from build123d import *

# Parameters (mm, degrees)
SKETCH1_W           = 25.4
SKETCH1_H           = 38.1
BOSS_EXTRUDE1_DEPTH = 609.6
SHELL1_T            = -3.175
SKETCH2_R           = 2.38125
CUT_EXTRUDE1_DEPTH  = 611.426262951


with BuildPart() as part:
    # Sketch1 → Boss-Extrude1 (new body)
    with BuildSketch(Plane.XY):
        Rectangle(SKETCH1_W, SKETCH1_H)
    extrude(amount=BOSS_EXTRUDE1_DEPTH)

    # Shell1
    shell1_openings = [part.faces().sort_by_distance(p)[0] for p in [
        (0, 0, 609.6),
        (0, 0, 0),
    ]]
    offset(amount=SHELL1_T, openings=shell1_openings, kind=Kind.INTERSECTION)

    # Sketch2 → Cut-Extrude1 (cut, through all)
    with BuildSketch(Plane(origin=(12.7, 0, 0), x_dir=(0, 0, -1), z_dir=(1, 0, 0))):
        with Locations(Location((-44.45, 6.35, 0), (0, 0, 90))):
            Circle(SKETCH2_R)
        with Locations(Location((-63.5, 6.35, 0), (0, 0, 90))):
            Circle(SKETCH2_R)
    extrude(amount=-CUT_EXTRUDE1_DEPTH, mode=Mode.SUBTRACT)


solid = part.part
Verification items for the finished model (mm, model axes). A direction names the side the tool comes from. Round coordinates to 2 decimals unless told otherwise and drop trailing zeros. Loops run counter-clockwise (first coordinate to the right, second up) from the corner with the lowest first, then second, coordinate; pieces in that order, holes last. Notation, with made-up numbers: (44, 22) - (90, 22) arc R24 ccw to (90, 50) - close; hole circle Ø9 at (89.5, 7). An arc over 180 degrees is marked (long way). Use a Markdown table: item, result. Add a question column.
1. Access from +Z, -Z, +X, -X, +Y, -Y to the whole of each face (thin tool, end or side, straight path). Record for faces 4 (the face through (-9.525, 0, 301)), 5 (the face through (12.7, 0, 301)).
2. Section check A-A, the plane x = -1.75. Record the boundary of the cut face in (y, z) (3 decimals).
3. Thickness scan on probe 1 along Z at (x, y) = (-11.15, 6.35); probe 2 along Y at (x, z) = (-1, 365.5) (3 decimals); probe 3 along X at (y, z) = (-0.5, 467) (3 decimals). Record the ranges inside material, lowest first. Write a range as [from, to].
4. Release check for a two-part mould opening along Y. For faces 1 (the face through (0, 15.875, 301)), 2 (the face through (0, 19.05, 301)), 3 (the face through (11, 0, 0)) record: released by +Y, released by -Y, zero draft, split by the parting line, or undercut.
5. Section check B-B, the plane z = 115. Record the boundary of the cut face in (x, y) (3 decimals).
6. Gauge pin test, flat end, axial feed: pin 1 (5.5 mm diameter, centred on y = 6.35, z = 44.45, fed in from +X). Record the tip position at first contact, or that the pin passes through.
Checks:
| question | item | result |
|---|---|---|
| 1 | face 4 | +Z, -Z |
| 1 | face 5 | +Z, -Z, +X, +Y, -Y |
| 2 | outline | (-19.05, 0) - (-15.875, 0) - (-15.875, 609.6) - (-19.05, 609.6) - close; (15.875, 0) - (19.05, 0) - (19.05, 609.6) - (15.875, 609.6) - close |
| 3 | probe 1 | z = [0, 42.07], [46.83, 61.12], [65.88, 609.6] |
| 3 | probe 2 | y = [-19.05, -15.875], [15.875, 19.05] |
| 3 | probe 3 | x = [-12.7, -9.525], [9.525, 12.7] |
| 4 | face 1 | undercut |
| 4 | face 2 | released by +Y |
| 4 | face 3 | zero draft |
| 5 | outline | (-12.7, -19.05) - (12.7, -19.05) - (12.7, 19.05) - (-12.7, 19.05) - close; hole (-9.525, -15.875) - (9.525, -15.875) - (9.525, 15.875) - (-9.525, 15.875) - close |
| 6 | pin 1 | stops at x = 12.7 |
